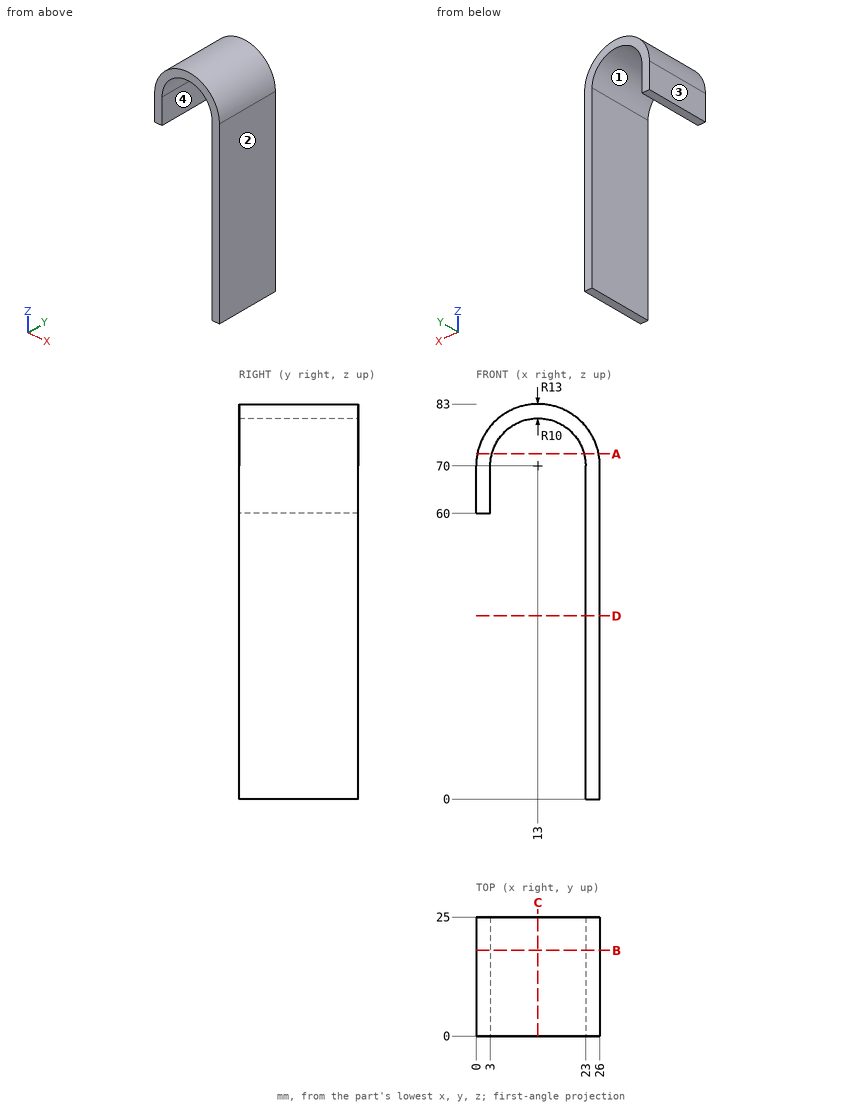
Print and shaded views of the part. All mm, measured from the part's lowest x, y and z. Give positions to 0.01 mm unless a question says otherwise; leave off trailing zeros. Loops run counter-clockwise (first coordinate to the right, second up) from the corner with the lowest first, then second, coordinate; pieces in that order, holes last. Notation, with made-up numbers: M 46,25 L 83,25 A28 cw 83,57 Z; hole C 81.5,56.5 d9. An arc over 180 degrees is marked long. Write each question's results on one line, items separated by ' | '.
Q1. Mould opens along X. For the marked faces 1, 2, 3 and 4 say: pulls with the +X half, pulls with the -X half, needs draft (parallel to the pull), parting line crosses it, or undercut.
Geometry check:
face 1: undercut | face 2: pulls with the +X half | face 3: pulls with the -X half | face 4: undercut
Q2. Flat gauge pins, fed straight in: P1, Ø3.5, axis at x = 1, y = 12, coming from the -Z side; P2, Ø3, axis at x = 7.5, y = 16.5, coming from the +Z side; P3, Ø1.5, axis at x = 7.5, y = 21.5, coming from the +Z side. Where does each tip first touch, or does it go through?
Geometry check:
P1: stops at z = 60 | P2: stops at z = 82.37 | P3: stops at z = 82.1
Q3. Band-saw the part on B-B on y = 18. Write the cut outline in (x, z), and give its area (3 significant figures).
Geometry check:
outline: M 0,60 L 3,60 L 3,70 A10 cw 23,70 L 23,0 L 26,0 L 26,70 A13 ccw 0,70 Z | area: 348 mm²
Q4. Band-saw the part on D-D on z = 38.5. Write the cut outline in (x, y), and give its area (3 significant figures).
Geometry check:
outline: M 23,0 L 26,0 L 26,25 L 23,25 Z | area: 75.0 mm²
Q5. Band-saw the part on C-C on x = 13. Write the cut outline in (y, z).
Geometry check:
outline: M 0,80 L 25,80 L 25,83 L 0,83 Z
Q6. Band-saw the part on A-A on z = 72.5. Write the cut outline in (x, y).
Geometry check:
outline: M 0.24,0 L 3.32,0 L 3.32,25 L 0.24,25 Z; M 22.68,0 L 25.76,0 L 25.76,25 L 22.68,25 Z
Q7. Probe probe 1 along X at (y, z) = (8, 69.5); probe 2 along X at (y, z) = (22.25, 46); probe 3 along Z at (x, y) = (5.75, 5.75). List the from-to ranges inside material, lowest first.
Geometry check:
probe 1: x = 0 to 3, 23 to 26 | probe 2: x = 23 to 26 | probe 3: z = 76.89 to 80.79
